from build123d import *

# Parameters (mm, degrees)
CYLINDER006_R     = 25
CYLINDER006_DEPTH = 12.5
FILLET007_1_R     = 8
FILLET007_2_R     = 3


with BuildPart() as part:
    # Cylinder006 → Cylinder006 (new body)
    with BuildSketch(Plane.XZ):
        Circle(CYLINDER006_R)
    extrude(amount=CYLINDER006_DEPTH)

    # Fillet007 1
    fillet007_1_edges = [part.edges().sort_by_distance(p)[0] for p in [
        (-25, -12.5, 0),
    ]]
    fillet(fillet007_1_edges, radius=FILLET007_1_R)

    # Fillet007 2
    fillet007_2_edges = [part.edges().sort_by_distance(p)[0] for p in [
        (-25, 0, 0),
    ]]
    fillet(fillet007_2_edges, radius=FILLET007_2_R)


solid = part.part
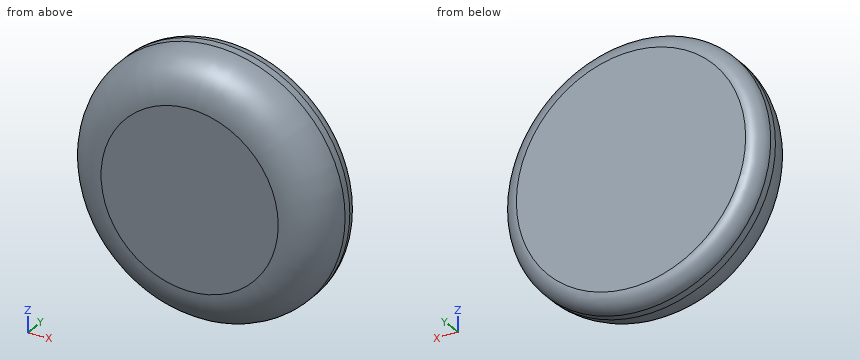
For this review, take the finished solid that the model builds, in its own axes (mm). Round coordinates to 2 decimals unless told otherwise and drop trailing zeros. Loops run counter-clockwise (first coordinate to the right, second up) from the corner with the lowest first, then second, coordinate; pieces in that order, holes last. Notation, with made-up numbers: (-32.75, -37) - (21.25, -37) arc R16 cw to (21.25, -24) - close; hole circle Ø4 at (-10, -23.75). An arc over 180 degrees is marked (long way). Put each result on its own line as item: value. Start each with the question number.
1. Consider section B-B on z = 0. State the section outline as (x, y) points.
2. Consider section C-C on y = -7. State the section outline as (x, z) points, plus the area to 3 significant figures.
3. Insertion check: P1, Ø6, axis at x = 10, y = -9, coming from the -Z side; P2, Ø4, axis at y = -6, z = 19.5, coming from the -X side; P3, Ø6, axis at x = 5.5, y = -7, coming from the -Z side. Each pin has a flat end and moves straight along its axis. Give the tip position at first contact, or say it passes through.
4. Consider section A-A on x = 0. State the section outline as (y, z) points, plus the area to 3 significant figures.
5. Consider section D-D on y = -2. State the section outline as (x, z) points.
6. For probe 1 along Z at (x, y) = (-14, -8.25); probe 2 along X at (y, z) = (-9.75, 2.5); probe 3 along Z at (x, y) = (22.5, -1.5), list the stretches that pass through material, from the lowest coordinate up. Write a range as [from, to].
Result sheet:
1. outline: (-25, -4.5) arc R8 ccw to (-17, -12.5) - (17, -12.5) arc R8 ccw to (25, -4.5) - (25, -3) arc R3 ccw to (22, 0) - (-22, 0) arc R3 ccw to (-25, -3) - close
2. outline: circle Ø49.2 at (0, 0)
2. area: 1,900 mm^2
3. P1: z = -23.34
3. P2: x = -17.71
3. P3: z = -24.78
4. outline: (-12.5, -17) arc R8 ccw to (-4.5, -25) - (-3, -25) arc R3 ccw to (0, -22) - (0, 22) arc R3 ccw to (-3, 25) - (-4.5, 25) arc R8 ccw to (-12.5, 17) - close
4. area: 594 mm^2
5. outline: circle Ø49.66 at (0, 0)
6. probe 1: [-19.58, 19.58]
6. probe 2: [-22.9, 22.9]
6. probe 3: [-9.94, 9.94]
